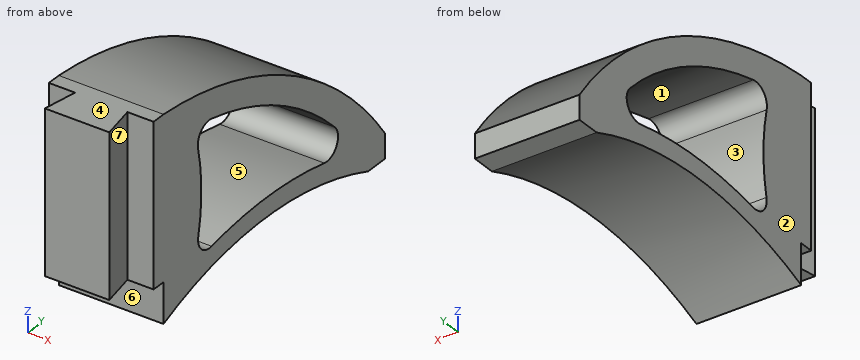
from build123d import *

# Parameters (mm, degrees)
BOSS_EXTRUDE2_DEPTH = 6.5
CUT_EXTRUDE1_DEPTH  = 47.778734485
CUT_EXTRUDE2_DEPTH  = 45.010875493


with BuildPart() as part:
    # Sketch2 → Boss-Extrude2 (new, symmetric)
    with BuildSketch(Plane(origin=(0, 0, 0), x_dir=(0, 0, -1), z_dir=(1, 0, 0))):
        with BuildLine():
            Line((-15.714870718, 0), (-15.714870718, -6))
            Line((-15.714870718, -6), (4.285129282, -6))
            Line((4.285129282, -6), (4.285129282, 0))
            Line((4.285129282, 0), (9.285129282, 0))
            ThreePointArc((9.285129282, 0), (5.701715974, 18), (9.285129282, 36))
            Line((9.285129282, 36), (9.285129282, 39))
            Line((9.285129282, 39), (6.285129282, 39))
            ThreePointArc((6.285129282, 39), (-9.226389961, 22.044959573), (-15.714870718, 0))
        make_face()
    extrude(amount=BOSS_EXTRUDE2_DEPTH, both=True)

    # Sketch3 → Cut-Extrude1 (cut, through all)
    with BuildSketch(Plane.XY.offset(15.714870718)):
        Polygon((6.5, -6), (6.5, -1.746538635), (3.25, -1.746538635), (4, -6), align=None)
        Polygon((-6.5, -6), (-4, -6), (-3.25, -1.746538635), (-6.5, -1.746538635), align=None)
    extrude(amount=-CUT_EXTRUDE1_DEPTH, mode=Mode.SUBTRACT)

    # Sketch4 → Cut-Extrude2 (cut, through all)
    with BuildSketch(Plane(origin=(6.5, 0, 0), x_dir=(0, 0, -1), z_dir=(1, 0, 0))):
        with BuildLine():
            ThreePointArc((4.293654014, 8.463820333), (3.356236623, 18.389014044), (4.406551478, 28.302896243))
            ThreePointArc((4.406551478, 28.302896243), (3.415993904, 30.4613018), (1.061425552, 30.151581393))
            ThreePointArc((1.061425552, 30.151581393), (-6.57340708, 20.201122888), (-10.929733391, 8.439970103))
            ThreePointArc((-10.929733391, 8.439970103), (-10.378680687, 6.611841621), (-8.545133867, 6.07909507))
            ThreePointArc((-8.545133867, 6.07909507), (-3.314593754, 6.65373917), (1.920364292, 6.120841452))
            ThreePointArc((1.920364292, 6.120841452), (3.736278671, 6.654920589), (4.293654014, 8.463820333))
        make_face()
    extrude(amount=-CUT_EXTRUDE2_DEPTH, mode=Mode.SUBTRACT)


solid = part.part
Can you work these out from the model? Positions are in its coordinate system, mm. Face numbers are marked on the shaded views. A direction names the side the tool comes from. Round coordinates to 2 decimals unless told otherwise and drop trailing zeros. Order: outer loops, then holes, each group sorted by start corner. A loop starts at its lowest first (then second) coordinate and runs counter-clockwise, first axis right, second up. Notation, with made-up numbers: M 44,68 L 100,68 A26 cw 100,89 Z; hole C -21,-4 d7. An arc over 180 degrees is marked long. Use a Markdown table: item, result.
1) Imagine slicing it at C-C (x = -1). List the corners of the cut face in (y, z) for me.
Geometry says:
| item | result |
|---|---|
| outline | M -6,-4.29 L 0,-4.29 L 0,-9.29 A47 cw 36,-9.29 L 39,-9.29 L 39,-6.29 A50.97 ccw 0,15.71 L -6,15.71 Z; hole M 6.08,8.55 A25 cw 6.12,-1.92 A2 ccw 8.46,-4.29 A50 cw 28.3,-4.41 A2 ccw 30.15,-1.06 A42 ccw 8.44,10.93 A2 ccw Z |
2) Imagine slicing it at D-D (z = 12). List the corners of the cut face in (x, y) for me, then the cut area to 3 significant figures.
Geometry says:
| item | result |
|---|---|
| outline | M -6.5,-1.75 L -3.25,-1.75 L -4,-6 L 4,-6 L 3.25,-1.75 L 6.5,-1.75 L 6.5,16.32 L -6.5,16.32 Z |
| area | 266 mm² |
3) On a 3-axis mill with a long thin cutter (end or side, diameter ignored), from which of +Z, -Z, +X, -X, +Y, -Y can I reach the whole of each face in a straight line? I mean the marked faces 5, 6 and 7. Say none if no direction works.
Geometry says:
| item | result |
|---|---|
| face 5 | +X, -X |
| face 6 | -Z, +X, -X, -Y |
| face 7 | +Z, -Z, +X |
4) If I drill on line 1 along Z through (x, y) = (-2.75, 18); line 2 along Y through (x, z) = (-1.25, 5.5); line 3 along Y through (x, z) = (-2.25, 7.5), over which ranges is the centre line in solid material (lowest first)?
Geometry says:
| item | result |
|---|---|
| line 1 | z = -5.7 to -3.36, 7.71 to 11.28 |
| line 2 | y = -6 to 6.55, 22.03 to 27.73 |
| line 3 | y = -6 to 6.28, 18.42 to 24.88 |
5) I'm going to push flat-ended pins straight in: P1, Ø2.5, axis at x = -0.5, z = -6.5, coming from the -Y side; P2, Ø1.5, axis at x = -0.5, y = 11, coming from the +Z side; P3, Ø6, axis at x = -0.5, y = 19.5, coming from the +Z side. Where does each tip first touch, or does it pass through?
Geometry says:
| item | result |
|---|---|
| P1 | stops at y = 0 |
| P2 | stops at z = 14.05 |
| P3 | stops at z = 11.93 |
6) Imagine slicing it at A-A (z = 5.25). List the corners of the cut face in (x, y) for me, then the cut area to 3 significant figures.
Geometry says:
| item | result |
|---|---|
| outline | M -6.5,-1.75 L -3.25,-1.75 L -4,-6 L 4,-6 L 3.25,-1.75 L 6.5,-1.75 L 6.5,6.57 L -6.5,6.57 Z; M -6.5,22.43 L 6.5,22.43 L 6.5,28.06 L -6.5,28.06 Z |
| area | 212 mm² |
7) Imagine slicing it at B-B (y = 26.5). List the corners of the cut face in (x, z) for me.
Geometry says:
| item | result |
|---|---|
| outline | M -6.5,-6.48 L 6.5,-6.48 L 6.5,-4.07 L -6.5,-4.07 Z; M -6.5,2.31 L 6.5,2.31 L 6.5,6.4 L -6.5,6.4 Z |
8) If we mould it in two halves opening along Z, with no side actions, what happens to the marked faces 1, 2, 3 and 4? For each: +Z half, -Z half, draft (parallel to the pull), parting line (faces both ways), or undercut.
Geometry says:
| item | result |
|---|---|
| face 1 | undercut |
| face 2 | draft |
| face 3 | undercut |
| face 4 | +Z half |
